Autodesk Inventor part; units mm, degrees
ref_plane "bracket_to_dummy_XY" through (0, 0, 0) normal (0, 1, 0) x (1, 0, 0)
ref_plane "bracket_to_dummy_YZ" through (0, 0, 0) normal (1, 0, 0) x (0, 0, -1)
ref_plane "bracket_to_dummy_ZX" through (0, 0, 0) normal (0, 0, -1) x (0, 1, 0)
sketch "Sketch_1" plane through (0, 0, 0) normal (1, 0, 0) x (0, 1, 0)
  line L0 (4, 35) -> (1, 35)
  arc A0 (1, 35) -> (0, 34) centre (1, 34) ccw
  line L1 (0, 34) -> (0, 1)
  arc A1 (0, 1) -> (1, 0) centre (1, 1) ccw
  line L2 (1, 0) -> (34, 0)
  arc A2 (34, 0) -> (35, 1) centre (34, 1) ccw
  line L3 (35, 1) -> (35, 4)
  arc A3 (35, 4) -> (34, 5) centre (34, 4) ccw
  line L4 (34, 5) -> (17.4142, 5)
  arc A4 (16.7071, 5.2929) -> (17.4142, 5) centre (17.4142, 6) ccw
  line L5 (16.7071, 5.2929) -> (14.878, 7.122)
  arc A5 (14.9333, 8.5874) -> (14.878, 7.122) centre (15.5851, 7.8291) ccw
  arc A6 (14.9333, 8.5874) -> (16.4188, 12.8512) centre (12, 12) ccw
  arc A7 (16.4188, 12.8512) -> (16.0465, 13.0843) centre (16.1242, 12.7945) ccw
  line L6 (16.0465, 13.0843) -> (14.3, 12.6163)
  arc A8 (14.3, 12.6163) -> (14.0805, 12.2857) centre (14.3777, 12.3265) ccw
  arc A9 (12.2857, 14.0805) -> (14.0805, 12.2857) centre (12, 12) ccw
  arc A10 (12.2857, 14.0805) -> (12.6163, 14.3) centre (12.3265, 14.3777) ccw
  line L7 (12.6163, 14.3) -> (13.0843, 16.0465)
  arc A11 (13.0843, 16.0465) -> (12.8512, 16.4188) centre (12.7945, 16.1242) ccw
  arc A12 (12.8512, 16.4188) -> (8.5874, 14.9333) centre (12, 12) ccw
  arc A13 (7.122, 14.878) -> (8.5874, 14.9333) centre (7.8291, 15.5851) ccw
  line L8 (7.122, 14.878) -> (5.2929, 16.7071)
  arc A14 (5, 17.4142) -> (5.2929, 16.7071) centre (6, 17.4142) ccw
  line L9 (5, 17.4142) -> (5, 34)
  arc A15 (5, 34) -> (4, 35) centre (4, 34) ccw
extrude "Extrusion1" add sketch "Sketch_1" along normal mid plane 14
sketch "Sketch_2" plane through (0, 0, 0) normal (0, 0, 1) x (1, 0, 0)
  circle A0 centre (0, 25) radius 2.75
extrude "Extrusion2" cut sketch "Sketch_2" along normal mid plane 10
sketch "Sketch_3" plane through (0, 0, 0) normal (0, 1, 0) x (-1, 0, 0)
  circle A0 centre (0, 25) radius 2.75
extrude "Extrusion3" cut sketch "Sketch_3" along normal mid plane 10
ref_plane "bracket_to_dummy_XY" through (0, 0, 0) normal (0, 1, 0) x (1, 0, 0)
ref_plane "bracket_to_dummy_YZ" through (0, 0, 0) normal (1, 0, 0) x (0, 0, -1)
ref_plane "bracket_to_dummy_ZX" through (0, 0, 0) normal (0, 0, -1) x (0, 1, 0)
ref_plane "to_bolt_1_6_XY" through (0, 25, 5) normal (0, 0, 1) x (1, 0, 0)
ref_plane "to_bolt_1_6_YZ" through (0, 25, 5) normal (1, 0, 0) x (0, 1, 0)
ref_plane "to_bolt_1_6_ZX" through (0, 25, 5) normal (0, 1, 0) x (0, 0, 1)
ref_plane "to_bolt_1_6_base_XY" through (0, 5, 25) normal (0, 1, 0) x (1, 0, 0)
ref_plane "to_bolt_1_6_base_YZ" through (0, 5, 25) normal (1, 0, 0) x (0, 0, -1)
ref_plane "to_bolt_1_6_base_ZX" through (0, 5, 25) normal (0, 0, -1) x (0, 1, 0)
ref_plane "to_nut_1_6_XY" through (0, 25, -2) normal (0, 0, 1) x (1, 0, 0)
ref_plane "to_nut_1_6_YZ" through (0, 25, -2) normal (1, 0, 0) x (0, 1, 0)
ref_plane "to_nut_1_6_ZX" through (0, 25, -2) normal (0, 1, 0) x (0, 0, 1)
ref_plane "to_nut_1_6_base_XY" through (0, -2, 25) normal (0, 1, 0) x (1, 0, 0)
ref_plane "to_nut_1_6_base_YZ" through (0, -2, 25) normal (1, 0, 0) x (0, 0, -1)
ref_plane "to_nut_1_6_base_ZX" through (0, -2, 25) normal (0, 0, -1) x (0, 1, 0)
ref_plane "to_screw_XY" through (0, 5, 25) normal (0, 1, 0) x (1, 0, 0)
ref_plane "to_screw_YZ" through (0, 5, 25) normal (1, 0, 0) x (0, 0, -1)
ref_plane "to_screw_ZX" through (0, 5, 25) normal (0, 0, -1) x (0, 1, 0)
ref_plane "to_screw10_XY" through (0, 5, 25) normal (0, 1, 0) x (1, 0, 0)
ref_plane "to_screw10_YZ" through (0, 5, 25) normal (1, 0, 0) x (0, 0, -1)
ref_plane "to_screw10_ZX" through (0, 5, 25) normal (0, 0, -1) x (0, 1, 0)
ref_plane "to_screw2_XY" through (0, 5, 25) normal (0, 1, 0) x (1, 0, 0)
ref_plane "to_screw2_YZ" through (0, 5, 25) normal (1, 0, 0) x (0, 0, -1)
ref_plane "to_screw2_ZX" through (0, 5, 25) normal (0, 0, -1) x (0, 1, 0)
ref_plane "to_screw3_XY" through (0, 25, 5) normal (0, 0, 1) x (1, 0, 0)
ref_plane "to_screw3_YZ" through (0, 25, 5) normal (1, 0, 0) x (0, 1, 0)
ref_plane "to_screw3_ZX" through (0, 25, 5) normal (0, 1, 0) x (0, 0, 1)
ref_plane "to_screw4_XY" through (0, 25, 5) normal (0, 0, 1) x (1, 0, 0)
ref_plane "to_screw4_YZ" through (0, 25, 5) normal (1, 0, 0) x (0, 1, 0)
ref_plane "to_screw4_ZX" through (0, 25, 5) normal (0, 1, 0) x (0, 0, 1)
ref_plane "to_screw5_XY" through (0, 5, 25) normal (0, 1, 0) x (1, 0, 0)
ref_plane "to_screw5_YZ" through (0, 5, 25) normal (1, 0, 0) x (0, 0, -1)
ref_plane "to_screw5_ZX" through (0, 5, 25) normal (0, 0, -1) x (0, 1, 0)
ref_plane "to_screw6_XY" through (0, 5, 25) normal (0, 1, 0) x (1, 0, 0)
ref_plane "to_screw6_YZ" through (0, 5, 25) normal (1, 0, 0) x (0, 0, -1)
ref_plane "to_screw6_ZX" through (0, 5, 25) normal (0, 0, -1) x (0, 1, 0)
ref_plane "to_screw7_XY" through (0, 25, 5) normal (0, 0, 1) x (1, 0, 0)
ref_plane "to_screw7_YZ" through (0, 25, 5) normal (1, 0, 0) x (0, 1, 0)
ref_plane "to_screw7_ZX" through (0, 25, 5) normal (0, 1, 0) x (0, 0, 1)
ref_plane "to_screw8_XY" through (0, 25, 5) normal (0, 0, 1) x (1, 0, 0)
ref_plane "to_screw8_YZ" through (0, 25, 5) normal (1, 0, 0) x (0, 1, 0)
ref_plane "to_screw8_ZX" through (0, 25, 5) normal (0, 1, 0) x (0, 0, 1)
ref_plane "to_screw9_XY" through (0, 25, 5) normal (0, 0, 1) x (1, 0, 0)
ref_plane "to_screw9_YZ" through (0, 25, 5) normal (1, 0, 0) x (0, 1, 0)
ref_plane "to_screw9_ZX" through (0, 25, 5) normal (0, 1, 0) x (0, 0, 1)
properties part number "NBLTS5_b"
Geometry check sheet. Reference: the model listing, model coordinates, mm. A direction names the side the tool comes from. Give positions to 0.01 mm unless a question says otherwise; leave off trailing zeros. Loops run counter-clockwise (first coordinate to the right, second up) from the corner with the lowest first, then second, coordinate; pieces in that order, holes last. Notation, with made-up numbers: (12.5, 46.25) - (56.5, 46.25) arc R28 ccw to (56.5, 65.25) - close; hole circle Ø5 at (75.25, -23). An arc over 180 degrees is marked (long way). Use CSV: the item, a comma, the result in double quotes. Start each with the question number.
Q1. Section check A-A, the plane y = 25. Record the cut outline in (x, z), and give its area (3 significant figures).
Q2. Scan lines: probe 1 along Y at (x, z) = (0, 2.5); probe 2 along Y at (x, z) = (1.5, 12). Record each from-to range of solid material in increasing order. Write a range as from..to.
Q3. Go/stop test with flat-tipped pins: pin 1 Ø7 at (x, y) = (0, 25) entering from +Z; pin 2 Ø5 at (x, z) = (0, 25) entering from -Y. Record where each tip stops, or that it passes through.
Q4. Access from +Z, -Z, +X, -X, +Y, -Y to the whole of each face (thin tool, end or side, straight path). Record for faces 4 (the face through (-0.098, 12.847, 15.161)), 5 (the face through (-0.098, 15.185, 12.854)), 6 (the face through (-2, 28, 5)), 7 (the face through (0, 0, 18)), 8 (the face through (0, 3, 35)).
Q5. Release check for a two-part mould opening along X. For faces 1 (the face through (-7, 9.6, 11.1)), 2 (the face through (-0.358, 22.273, 2.465)), 3 (the face through (0, 6, 16)) record: +X half, -X half, draft (parallel to the pull), parting line (faces both ways), or undercut.
Q6. Section check D-D, the plane x = 0. Count the separate pieces of the cut face and the enclosed holes in it, and give its area (3 significant figures).
Q7. Section check C-C, the plane y = 3. Record the cut outline in (x, z).
Findings below:
1,outline,"(-7, 0) - (-2.75, 0) - (-2.75, 5) - (-7, 5) - close; (2.75, 0) - (7, 0) - (7, 5) - (2.75, 5) - close"
1,area,"42.5 mm^2"
2,probe 1,"y = 0..22.25, 27.75..35"
2,probe 2,"y = 0..9.9, 14.1..16.5"
3,pin 1,"stops at z = 5"
3,pin 2,"passes through"
4,face 4,"+X, -X, +Y"
4,face 5,"+Z, +X, -X"
4,face 6,"+Z, +X, -X, +Y"
4,face 7,"+Z, -Z, +X, -X, -Y"
4,face 8,"+Z, +X, -X, +Y, -Y"
5,face 1,"-X half"
5,face 2,"undercut"
5,face 3,"draft"
6,separate pieces,"3"
6,enclosed holes,"0"
6,area,"364 mm^2"
7,outline,"(-7, 0) - (7, 0) - (7, 35) - (-7, 35) - close; hole circle Ø5.5 at (0, 25)"
